Here's the drawing with two shaded views (mm, measured from the low corner). I have some questions. Round coordinates to 2 decimals unless told otherwise and drop trailing zeros. Loops run counter-clockwise (first coordinate to the right, second up) from the corner with the lowest first, then second, coordinate; pieces in that order, holes last. Notation, with made-up numbers: (76, -13) -> (83, -13) arc R19 cw to (83, 9) -> close; hole circle Ø10 at (-24.75, 73.5). An arc over 180 degrees is marked (long way). Write each question's results on one line, items separated by ' | '.
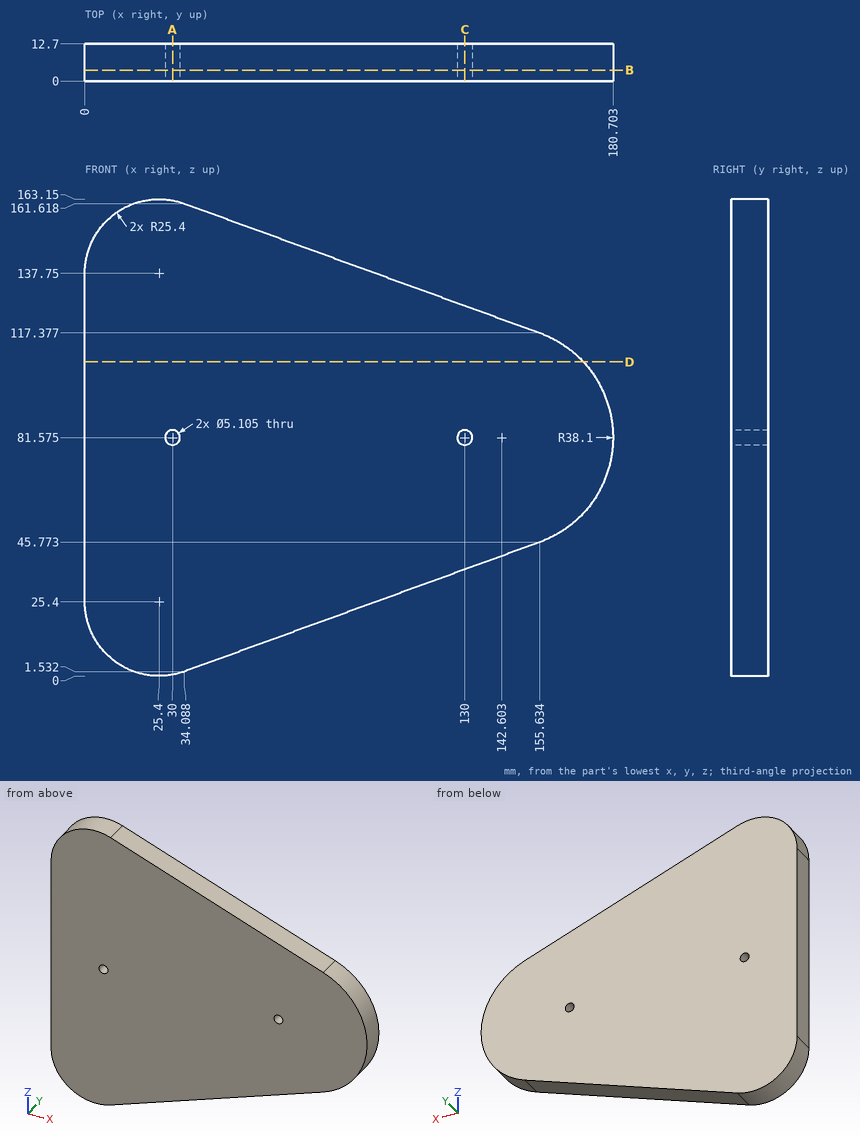
1. If we section it at B-B (y = 3.75): State how many separate pieces and enclosed holes the cut face has, then the cut area to 3 significant figures.
Final values:
separate pieces: 1 | enclosed holes: 2 | area: 20,600 mm2
2. If we section it at C-C (x = 130): List the corners of the cut face in (y, z) for me.
Final values:
outline: (0, 36.44) -> (12.7, 36.44) -> (12.7, 79.02) -> (0, 79.02) -> close; (0, 84.13) -> (12.7, 84.13) -> (12.7, 126.71) -> (0, 126.71) -> close
3. If we section it at D-D (z = 107.5): List the corners of the cut face in (x, y) for me.
Final values:
outline: (0, 0) -> (170.52, 0) -> (170.52, 12.7) -> (0, 12.7) -> close
4. Please list where these lines run through material, in increasing order: line 1 (Z direction, x = 130, y = 8); line 2 (X direction, y = 9, z = 95.5); line 3 (X direction, y = 5, z = 92.5). Write a range as from..to.
Final values:
line 1: 36.44..79.02, 84.13..126.71 | line 2: 0..178.07 | line 3: 0..179.1
5. If we section it at A-A (x = 30): List the corners of the cut face in (y, z) for me.
Final values:
outline: (0, 0.42) -> (12.7, 0.42) -> (12.7, 79.02) -> (0, 79.02) -> close; (0, 84.13) -> (12.7, 84.13) -> (12.7, 162.73) -> (0, 162.73) -> close
6. Will these pins go through, and if not, where does the flat tip stop? pin 1 (3 mm diameter, centred on x = 53.5, z = 118, fed in from -Y); pin 2 (4 mm diameter, centred on x = 58.5, y = 8.5, fed in from -Z); pin 3 (6 mm diameter, centred on x = 18.5, y = 11, fed in from -Z); pin 4 (4 mm diameter, centred on x = 30, z = 81.575, fed in from +Y).
Final values:
pin 1: y = 0 | pin 2: z = 9.69 | pin 3: z = 0.3 | pin 4: through
